The listing builds one solid part. Answer for the finished solid, in the listing's coordinates (mm). Face numbers are marked on the shaded views. Round coordinates to 2 decimals unless told otherwise and drop trailing zeros. Write each loop counter-clockwise with the first axis right and the second up, starting at its lowest first coordinate (ties: lowest second). Pieces come first, ordered by that corner, then holes. Notation, with made-up numbers: (89, -29.75) - (142, -29.75) arc R38 ccw to (142, 9.25) - close; hole circle Ø6 at (-15, 69.25). An arc over 180 degrees is marked (long way). Answer in a Markdown table with one row per item.
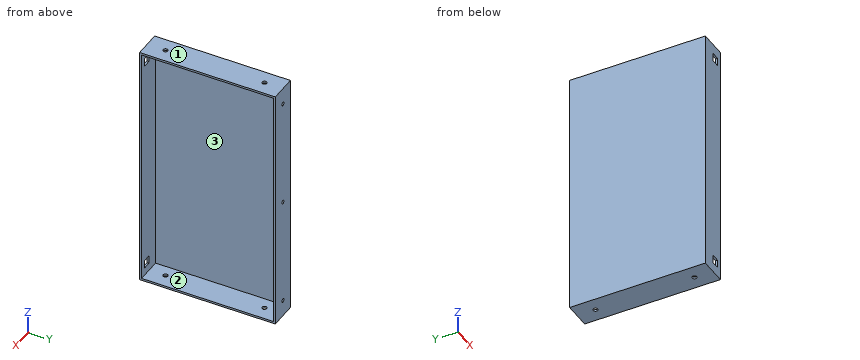
from build123d import *

# Parameters (mm, degrees)
F0_W     = 38.1
F0_H     = 187.325
F1_DEPTH = 171.45
F2_T     = -2.778125
F3_R     = 2.5796875
F4_DEPTH = 2.778125
F5_R     = 3.175
F6_DEPTH = 342.901
F7_W     = 11.1125
F7_H     = 11.1125
F8_DEPTH = 2.778125


# Not quite as in the source:
# - a feature names something its author has since deleted; it is built from what else it names


with BuildPart() as f1:
    # F0 (on Top) → F1 (new body, symmetric)
    with BuildSketch(Plane.XY):
        with Locations((19.05, 93.6625)):
            Rectangle(F0_W, F0_H)
    extrude(amount=F1_DEPTH, both=True)

    # F2
    f2_openings = [f1.faces().sort_by_distance(p)[0] for p in [
        (38.1, 93.6625, 0),
    ]]
    offset(amount=F2_T, openings=f2_openings)

    # F3 (on face) → F4 (cut, through all)
    with BuildSketch(Plane(origin=(0, 187.325, 0), x_dir=(-1, 0, 0), z_dir=(0, 1, 0))):
        with Locations((-19.05, 148.43125)):
            Circle(F3_R)
        with Locations((-19.05, 0)):
            Circle(F3_R)
        with Locations((-19.05, -148.43125)):
            Circle(F3_R)
    extrude(amount=-F4_DEPTH, mode=Mode.SUBTRACT)

    # F5 (on face) → F6 (cut, through all)
    with BuildSketch(Plane.XY.offset(171.45)):
        with Locations((19.05, 161.925)):
            Circle(F5_R)
        with Locations((19.05, 25.4)):
            Circle(F5_R)
    extrude(amount=-F6_DEPTH, mode=Mode.SUBTRACT)

    # F7 (on face) → F8 (cut, through all)
    with BuildSketch(Plane.XZ):
        with Locations((25.4, 152.4)):
            Rectangle(F7_W, F7_H)
        with Locations((25.4, -152.4)):
            Rectangle(F7_W, F7_H)
    extrude(amount=-F8_DEPTH, mode=Mode.SUBTRACT)


solid = f1.part
(1) Section B-B (x = 34.5) is taken. Give the vertices of the cut face in (y, z) (3 decimals).
Checked values:
| item | result |
|---|---|
| outline | (0, -171.45) - (187.325, -171.45) - (187.325, 171.45) - (0, 171.45) - close; hole (2.778, -168.672) - (184.547, -168.672) - (184.547, 168.672) - (2.778, 168.672) - close |
(2) A flat-ended cylindrical pin translates along its axis: pin 1 (6 mm diameter, centred on x = 19.05, z = 148.43, fed in from -Y). Find the tip coordinate at first contact, or state that the pin passes through.
Checked values:
| item | result |
|---|---|
| pin 1 | stops at y = 0 |
(3) Section C-C (z = -20) is taken. Give the vertices of the cut face in (x, y) (3 decimals).
Checked values:
| item | result |
|---|---|
| outline | (0, 0) - (38.1, 0) - (38.1, 2.778) - (2.778, 2.778) - (2.778, 184.547) - (38.1, 184.547) - (38.1, 187.325) - (0, 187.325) - close |
(4) For a pull along Y with two mould halves and no side action, classify the marked faces 1, 2 and 3 as pulls with the +Y half, pulls with the -Y half, needs draft (parallel to the pull), parting line crosses it, or undercut.
Checked values:
| item | result |
|---|---|
| face 1 | needs draft |
| face 2 | undercut |
| face 3 | undercut |
(5) Find the intervals of material crossed by line 1 (Z direction, x = 19.05, y = 186); line 2 (Z direction, x = 20.5, y = 175); line 3 (Y direction, x = 19.05, z = -169.85) (3 decimals), in increasing order.
Checked values:
| item | result |
|---|---|
| line 1 | z = -171.45 to -151.01, -145.85 to -2.58, 2.58 to 145.85, 151.01 to 171.45 |
| line 2 | z = -171.45 to -168.67, 168.67 to 171.45 |
| line 3 | y = 0 to 22.225, 28.575 to 158.75, 165.1 to 187.325 |
(6) Section A-A (y = 25.4) is taken. Give the vertices of the cut face in (x, z) (3 decimals).
Checked values:
| item | result |
|---|---|
| outline | (0, -171.45) - (15.875, -171.45) - (15.875, -168.672) - (2.778, -168.672) - (2.778, 168.672) - (15.875, 168.672) - (15.875, 171.45) - (0, 171.45) - close; (22.225, -171.45) - (38.1, -171.45) - (38.1, -168.672) - (22.225, -168.672) - close; (22.225, 168.672) - (38.1, 168.672) - (38.1, 171.45) - (22.225, 171.45) - close |
(7) Section D-D (y = 73) is taken. Give the vertices of the cut face in (x, z).
Checked values:
| item | result |
|---|---|
| outline | (0, -171.45) - (38.1, -171.45) - (38.1, -168.67) - (2.78, -168.67) - (2.78, 168.67) - (38.1, 168.67) - (38.1, 171.45) - (0, 171.45) - close |
